```python
from build123d import *

# Parameters (mm, degrees)
SKETCH1_W                       = 5.5
SKETCH1_H                       = 4
SKETCH2_R                       = 2.5
BOSS_EXTRUDE1_DEPTH             = 5
SKETCH3_R                       = 2.95
BOSS_EXTRUDE2_DEPTH             = 5.9
F_2_0_2_DIAMETER_HOLE1_D        = 2
TAP_DRILL_FOR_M3X0_5_TAP1_D     = 2.5
TAP_DRILL_FOR_M3X0_5_TAP1_DEPTH = 6
TAP_DRILL_FOR_M3X0_5_TAP1_TIP   = 0.751075774
CHAMFER1_SIZE                   = 0.5
CHAMFER2_SIZE                   = 0.133974596
CHAMFER2_SIZE2                  = 0.5


with BuildPart() as part:
    # Sketch1 → Revolve1 (revolve)
    with BuildSketch(Plane.XY, mode=Mode.PRIVATE) as revolve1_sk:
        with Locations((7.75, 2)):
            Rectangle(SKETCH1_W, SKETCH1_H)
    revolve(revolve1_sk.sketch.rotate(Axis((5, 0, 0), (1, 0, 0)), 270), axis=Axis((5, 0, 0), (1, 0, 0)))

    # Sketch2 → Boss-Extrude1 (add)
    with BuildSketch(Plane.ZY.offset(-5)):
        Circle(SKETCH2_R)
    extrude(amount=BOSS_EXTRUDE1_DEPTH)

    # Sketch3 → Boss-Extrude2 (add)
    with BuildSketch(Plane(origin=(10.5, 0, 0), x_dir=(0, 0, -1), z_dir=(1, 0, 0))):
        Circle(SKETCH3_R)
    extrude(amount=BOSS_EXTRUDE2_DEPTH)

    # Ø2.0 (2) Diameter Hole1 (through all)
    with Locations(Plane(origin=(8, -4, 0), x_dir=(0, 0, -1), z_dir=(0, -1, 0))):
        with Locations((0, 0)):
            Hole(F_2_0_2_DIAMETER_HOLE1_D / 2)

    # Tap Drill for M3x0.5 Tap1
    with Locations(Plane(origin=(16.4, 0, 0), x_dir=(0, 0, -1), z_dir=(1, 0, 0))):
        with Locations((0, 0)):
            Hole(TAP_DRILL_FOR_M3X0_5_TAP1_D / 2, depth=TAP_DRILL_FOR_M3X0_5_TAP1_DEPTH)
            with Locations((0, 0, -(TAP_DRILL_FOR_M3X0_5_TAP1_DEPTH + TAP_DRILL_FOR_M3X0_5_TAP1_TIP / 2))):  # 118° drill point
                Cone(0, TAP_DRILL_FOR_M3X0_5_TAP1_D / 2, TAP_DRILL_FOR_M3X0_5_TAP1_TIP, mode=Mode.SUBTRACT)

    # Chamfer1
    chamfer1_edges = [part.edges().sort_by_distance(p)[0] for p in [
        (0, 0, -2.5),
    ]]
    chamfer(chamfer1_edges, length=CHAMFER1_SIZE)

    # Chamfer2
    chamfer2_edges = [part.edges().sort_by_distance(p)[0] for p in [
        (5, 0, 4),
    ]]
    chamfer2_side = [part.faces().sort_by_distance(p)[0] for p in [
        (5, 0, 3.886862915),
    ]]
    chamfer(chamfer2_edges, length=CHAMFER2_SIZE, length2=CHAMFER2_SIZE2, reference=chamfer2_side[0])


solid = part.part
```
Work out the finished part from the listing and answer in its coordinate system (mm). A direction names the side the tool comes from. Give positions to 0.01 mm unless a question says otherwise; leave off trailing zeros. Order: outer loops, then holes, each group sorted by start corner. A loop starts at its lowest first (then second) coordinate and runs counter-clockwise, first axis right, second up. Notation, with made-up numbers: (-19.5, 86) - (-1.5, 86) arc R31 ccw to (-1.5, 124) - close; hole circle Ø4 at (48.5, 13.25). An arc over 180 degrees is marked (long way). One line per item, written item: value. Start each with the question number.
1. Section A-A, the plane x = 12.5 is taken. Write down the section's boundary in (y, z).
2. Each of these flat-tipped pins is pushed along its axis until it touches: pin 1 Ø2 at (y, z) = (0, 0) entering from +X; pin 2 Ø4 at (x, y) = (10, -3) entering from -Z. Where does it stop, or does it pass through?
3. Section B-B, the plane x = 8 is taken. Write down the section's boundary in (y, z), then the cut area to 3 significant figures.
4. Which of the six approach directions +Z, -Z, +X, -X, +Y, -Y give full straight-line access (tool end or side, diameter ignored) to faces 4 (the face through (8.035, -3.549, -1.846)), 5 (the face through (5, -3, 0)), 6 (the face through (13.409, 0.13, 2.947))?
5. Consider line 1 (Y direction, x = 14.8, z = 0); line 2 (X direction, y = -0.5, z = -2.5); line 3 (X direction, y = 2, z = -0.5). Determine where each line is inside the solid, lowest interval first.
6. For a pull along Z with two mould halves and no side action, classify faces 1 (the face through (2.78, -2.44, -0.54)), 2 (the face through (9, 0, 0)), 3 (the face through (16.4, -1, -1)) as released by +Z, released by -Z, zero draft, split by the parting line, or undercut.
7. Section C-C, the plane x = 3 is taken. Write down the section's boundary in (y, z).
Filled sheet:
1. outline: circle Ø5.9 at (0, 0); hole circle Ø2.5 at (0, 0)
2. pin 1: x = 10.25
2. pin 2: z = -3.87
3. outline: (-3.87, -1) arc R4 ccw to (3.87, -1) - close; (-3.87, 1) - (3.87, 1) arc R4 ccw to start
3. area: 34.4 mm²
4. face 4: +X, -X
4. face 5: -X
4. face 6: +X
5. line 1: -2.95 to -1.25, 1.25 to 2.95
5. line 2: 5 to 16.4
5. line 3: 0.06 to 7.13, 8.87 to 16.4
6. face 1: split by the parting line
6. face 2: undercut
6. face 3: zero draft
7. outline: circle Ø5 at (0, 0)
